Here's how the part is built. I have some questions about the finished solid (model axes, mm). Face numbers are marked on the shaded views. A direction names the side the tool comes from. Give positions to 0.01 mm unless a question says otherwise; leave off trailing zeros. Loops run counter-clockwise (first coordinate to the right, second up) from the corner with the lowest first, then second, coordinate; pieces in that order, holes last. Notation, with made-up numbers: (-13, -34) - (12, -34) arc R13 cw to (12, -14) - close; hole circle Ø8 at (42, 2.5). An arc over 180 degrees is marked (long way). Use one line per item in the form item = value.
from build123d import *

# Parameters (mm, degrees)
F1_DEPTH = 70
F2_R     = 5
F3_DEPTH = 25
F4_R     = 2


with BuildPart() as f1:
    # F0 (on Top) → F1 (new body)
    with BuildSketch(Plane.XY):
        with BuildLine():
            Line((-17.657248, -31.933628), (-17.657248, 61.409633))
            Line((-17.657248, 61.409633), (-22.657248, 61.409633))
            Line((-22.657248, 61.409633), (-22.657248, -31.933628))
            ThreePointArc((-22.657248, -31.933628), (-24.080087, -34.4856), (-26.998956, -34.616876))
            Line((-26.998956, -34.616876), (-59.862951, -18.183851))
            Line((-59.862951, -18.183851), (-62.09913, -22.655931))
            Line((-62.09913, -22.655931), (-17.37833, -45.017729))
            Line((-17.37833, -45.017729), (-1.489394, -30.969989))
            ThreePointArc((-1.489394, -30.969989), (1.340461, -27.130205), (2.342752, -22.466792))
            Line((2.342752, -22.466792), (2.342752, -15.403016))
            Line((2.342752, -15.403016), (-2.657248, -15.403016))
            Line((-2.657248, -15.403016), (-2.657248, -22.466792))
            ThreePointArc((-2.657248, -22.466792), (-3.218001, -25.075838), (-4.801224, -27.224087))
            Line((-4.801224, -27.224087), (-12.67015, -34.181169))
            ThreePointArc((-12.67015, -34.181169), (-15.889868, -34.668705), (-17.657248, -31.933628))
        make_face()
    extrude(amount=F1_DEPTH)

    # F2 (on face) → F3 (cut)
    with BuildSketch(Plane.YZ.offset(-17.657248)):
        with Locations((46.409633, 55)):
            Circle(F2_R)
        with Locations((46.409633, 35)):
            Circle(F2_R)
        with Locations((46.409633, 15)):
            Circle(F2_R)
        with Locations((26.409633, 55)):
            Circle(F2_R)
        with Locations((26.409633, 35)):
            Circle(F2_R)
        with Locations((26.409633, 15)):
            Circle(F2_R)
        with Locations((6.409633, 55)):
            Circle(F2_R)
        with Locations((6.409633, 35)):
            Circle(F2_R)
        with Locations((6.409633, 15)):
            Circle(F2_R)
        with Locations((-13.590367, 55)):
            Circle(F2_R)
        with Locations((-13.590367, 35)):
            Circle(F2_R)
        with Locations((-13.590367, 15)):
            Circle(F2_R)
    extrude(amount=-F3_DEPTH, mode=Mode.SUBTRACT)

    # F4
    f4_edges = [f1.edges().sort_by_distance(p)[0] for p in [
        (-17.37833, -45.017729, 35),
    ]]
    fillet(f4_edges, radius=F4_R)


solid = f1.part
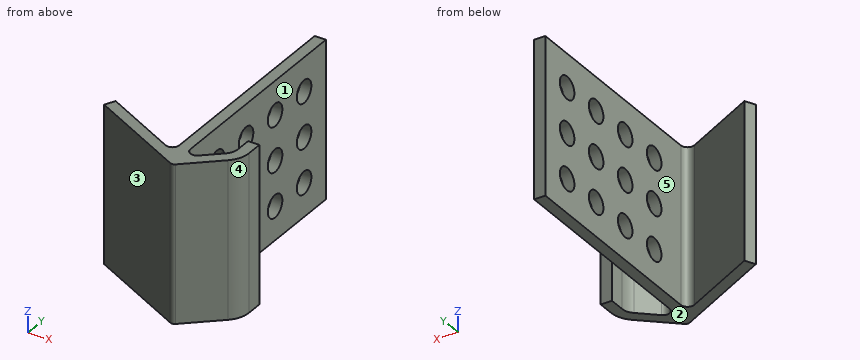
(1) Thinking about a two-plate mould opening in X: for the marked faces 1, 2 and 3, which applies, pulls with the +X half, pulls with the -X half, needs draft (parallel to the pull), parting line crosses it, or undercut?
Geometry says:
face_1 = undercut
face_2 = needs draft
face_3 = pulls with the -X half
(2) If we section it at A-A (z = 15): Give the number of separate pieces and of enclosed holes in the cut face, plus the area to 3 significant figures.
Geometry says:
separate_pieces = 5
enclosed_holes = 0
area = 724 mm²
(3) If we section it at D-D (y = -14): List the corners of the cut face in (x, z) for me, plus the area to 3 significant figures.
Geometry says:
outline = (-22.66, 0) - (-17.66, 0) - (-17.66, 10.02) - (-22.66, 10.02) - close; (-22.66, 19.98) - (-17.66, 19.98) - (-17.66, 30.02) - (-22.66, 30.02) - close; (-22.66, 39.98) - (-17.66, 39.98) - (-17.66, 50.02) - (-22.66, 50.02) - close; (-22.66, 59.98) - (-17.66, 59.98) - (-17.66, 70) - (-22.66, 70) - close
area = 201 mm²
(4) If we section it at C-C (z = 42): List the corners of the cut face in (x, y) for me, plus the area to 3 significant figures.
Geometry says:
outline = (-62.1, -22.66) - (-18.59, -44.41) arc R2 ccw to (-16.37, -44.12) - (-1.49, -30.97) arc R11.35 ccw to (2.34, -22.47) - (2.34, -15.4) - (-2.66, -15.4) - (-2.66, -22.47) arc R6.35 cw to (-4.8, -27.22) - (-12.67, -34.18) arc R3 cw to (-17.66, -31.93) - (-17.66, 61.41) - (-22.66, 61.41) - (-22.66, -31.93) arc R3 cw to (-27, -34.62) - (-59.86, -18.18) - close
area = 924 mm²
(5) For the marked faces 4 and 5, which set-ups out of +Z, -Z, +X, -X, +Y, -Y let a thin tool reach every point of the face, with its end or its side?
Geometry says:
face_4 = +Z, -Z, +X, -Y
face_5 = +Z, -Z, +Y
(6) If I drill on probe 1 along X at (y, z) = (-20.5, 24.5); probe 2 along X at (y, z) = (-33, 58); probe 3 along X at (y, z) = (-15.5, 43.5), over which ranges is the centre line in solid material (lowest first)?
Geometry says:
probe_1 = -61.02 to -55.23, -22.66 to -17.66, -2.66 to 2.34
probe_2 = -41.41 to -30.23, -22.85 to -17.46, -11.33 to -3.79
probe_3 = -22.66 to -17.66, -2.66 to 2.34
(7) For P1, Ø12, axis at x = -4.5, z = 38, coming from the -Y side; P2, Ø1, axis at x = -42, z = 30, coming from the +Y side; P3, Ø21, axis at y = 17.5, z = 33, coming from the -X side, each with a flat end and sliding along its axis, tell me the tip position at first contact or that it passes through.
Geometry says:
P1 = -38.94
P2 = -26.87
P3 = -22.66
(8) If we section it at B-B (y = -29.5): List the corners of the cut face in (x, z) for me, plus the area to 3 significant figures.
Geometry says:
outline = (-48.41, 0) - (-37.23, 0) - (-37.23, 70) - (-48.41, 70) - close; (-22.66, 0) - (-17.66, 0) - (-17.66, 70) - (-22.66, 70) - close; (-7.38, 0) - (-0.1, 0) - (-0.1, 70) - (-7.38, 70) - close
area = 1,640 mm²
